For this review, take the finished solid that the model builds, in its own axes (mm). A direction names the side the tool comes from. Round coordinates to 2 decimals unless told otherwise and drop trailing zeros. Order: outer loops, then holes, each group sorted by start corner. A loop starts at its lowest first (then second) coordinate and runs counter-clockwise, first axis right, second up. Notation, with made-up numbers: (16.25, 78) - (66.25, 78) arc R21 cw to (66.25, 108) - close; hole circle Ø10 at (-24, 87). An arc over 180 degrees is marked (long way). Write each question's results on one line, items separated by ' | '. Start each with the question number.
(1) Take a section at D-D, the plane y = -15.5. Give the boundary of the cut face in (x, z).
(2) Take a section at A-A, the plane z = 0. Give the number of separate pieces and of enclosed holes in the cut face, plus the area to 3 significant figures.
(3) Take a section at B-B, the plane x = 0. Give the boundary of the cut face in (y, z).
(4) Insertion check: pin 1 Ø4 at (x, z) = (11, 11.5) entering from +Y; pin 2 Ø8 at (x, z) = (29.5, -4) entering from -Y; pin 3 Ø10 at (x, z) = (31, -6) entering from +Y; pin 4 Ø12 at (y, z) = (12.5, 5.5) entering from -X. Each pin has a flat end and moves straight along its axis. Give the tip position at first contact, or say it passes through.
(5) Take a section at C-C, the plane y = 6.5. Give the boundary of the cut face in (x, z).
(6) For faces 5 (the flat face through (9, -12.5, 5)), 6 (the cylindrical face through (-1.099, -0.343, 24.976)), 7 (the cylindrical face through (45, 7, 0)), 8 (the flat face through (9, 12.5, -5)), 9 (the flat face through (17, 24.5, -13)), list the 3-axis set-ups (+Z, -Z, +X, -X, +Y, -Y) from which the entire face can be reached by the end or side of a thin tool; tool diameter is ignored.
(7) For L1, parallel to X at y = 16, z = 0; L2, parallel to Y at x = -16, z = -9.5; L3, parallel to Y at x = 27, z = 6, list the stretches that pass through material, from the lowest coordinate up. Write a range as from..to.
(8) Draft analysis for pull direction X (two halves, no side actions). For faces 1 (the cylindrical face through (22.26, 7.46, 13.64)), 2 (the cylindrical face through (8.96, 0.18, -4.66)), 3 (the cylindrical face through (-6.32, 18.58, -20.08)), 4 (the cylindrical face through (-22.26, 7.46, 13.64)), state which applies: pulls with the +X half, pulls with the -X half, needs draft (parallel to the pull), parting line crosses it, or undercut.
```python
from build123d import *

# Parameters (mm, degrees)
BOSS_EXTRUDE1_START = 5
SKETCH2_R           = 3.75
BOSS_EXTRUDE1_DEPTH = 5


with BuildPart() as part:
    # Sketch1 → Revolve1 (revolve)
    with BuildSketch(Plane.XY, mode=Mode.PRIVATE) as revolve1_sk:
        Polygon((21.05, 24.5), (25, 24.5), (25, -24.5), (21.05, -24.5), (21.05, -12.5), (10.1, -12.5), (10.1, 12.5), (21.05, 12.5), align=None)
    revolve(revolve1_sk.sketch.rotate(Axis((0, 0, 0), (0, 1, 0)), 90), axis=Axis((0, 0, 0), (0, 1, 0)))

    # Sketch2 → Boss-Extrude1 (add)
    # profile 1 of 2: a face of its own
    with BuildSketch(Plane(origin=(0, 0, 0), x_dir=(1, 0, 0), z_dir=(0, 1, 0)).offset(BOSS_EXTRUDE1_START)):
        with BuildLine():
            Line((-39.854181584, 7.12094299), (-26.911060299, 11.399934945))
            ThreePointArc((-26.911060299, 11.399934945), (-22.323138818, 13.598174791), (-18.438265476, 16.882842362))
            Line((-18.438265476, 16.882842362), (-18.438265476, -16.882842362))
            ThreePointArc((-18.438265476, -16.882842362), (-22.323138818, -13.598174791), (-26.911060299, -11.399934945))
            Line((-26.911060299, -11.399934945), (-39.854181584, -7.12094299))
            ThreePointArc((-39.854181584, -7.12094299), (-45, 0), (-39.854181584, 7.12094299))
        make_face()
        with Locations(Location((-37.5, 0, 0), (0, 0, 270))):
            Circle(SKETCH2_R, mode=Mode.SUBTRACT)
    # profile 2 of 2: a face of its own
    with BuildSketch(Plane(origin=(0, 0, 0), x_dir=(1, 0, 0), z_dir=(0, 1, 0)).offset(BOSS_EXTRUDE1_START)):
        with BuildLine():
            Line((18.438265476, 16.882842362), (18.438265476, -16.882842362))
            ThreePointArc((18.438265476, -16.882842362), (22.323138818, -13.598174791), (26.911060299, -11.399934945))
            Line((26.911060299, -11.399934945), (39.854181584, -7.12094299))
            ThreePointArc((39.854181584, -7.12094299), (45, 0), (39.854181584, 7.12094299))
            Line((39.854181584, 7.12094299), (26.911060299, 11.399934945))
            ThreePointArc((26.911060299, 11.399934945), (22.323138818, 13.598174791), (18.438265476, 16.882842362))
        make_face()
        with Locations(Location((37.5, 0, 0), (0, 0, 90))):
            Circle(SKETCH2_R, mode=Mode.SUBTRACT)
    extrude(amount=BOSS_EXTRUDE1_DEPTH)


solid = part.part
```
Results below:
1) outline: circle Ø50 at (0, 0); hole circle Ø42.1 at (0, 0)
2) separate pieces: 4 | enclosed holes: 0 | area: 1,060 mm^2
3) outline: (-24.5, -25) - (24.5, -25) - (24.5, -21.05) - (12.5, -21.05) - (12.5, -10.1) - (-12.5, -10.1) - (-12.5, -21.05) - (-24.5, -21.05) - close; (-24.5, 21.05) - (-12.5, 21.05) - (-12.5, 10.1) - (12.5, 10.1) - (12.5, 21.05) - (24.5, 21.05) - (24.5, 25) - (-24.5, 25) - close
4) pin 1: stops at y = 12.5 | pin 2: stops at y = 5 | pin 3: stops at y = 10 | pin 4: stops at x = -45
5) outline: (-39.85, -7.12) - (-26.91, -11.4) arc R20 cw to (-18.44, -16.88) arc R25 ccw to (18.44, -16.88) arc R20 cw to (26.91, -11.4) - (39.85, -7.12) arc R7.5 ccw to (39.85, 7.12) - (26.91, 11.4) arc R20 cw to (18.44, 16.88) arc R25 ccw to (-18.44, 16.88) arc R20 cw to (-26.91, 11.4) - (-39.85, 7.12) arc R7.5 ccw to start; hole circle Ø7.5 at (-37.5, 0); hole circle Ø20.2 at (0, 0); hole circle Ø7.5 at (37.5, 0)
6) face 5: -Y | face 6: none | face 7: +X, +Y, -Y | face 8: +Y | face 9: +Z, -Z, +X, -X, +Y
7) L1: x = -25..-21.05, 21.05..25 | L2: y = -12.5..12.5 | L3: y = 5..10
8) face 1: pulls with the +X half | face 2: undercut | face 3: undercut | face 4: pulls with the -X half
